For this review, take the finished solid that the model builds, in its own axes (mm). A direction names the side the tool comes from. Coordinates: 2 decimals unless noted, no trailing zeros. Write each loop counter-clockwise with the first axis right and the second up, starting at its lowest first coordinate (ties: lowest second). Pieces come first, ordered by that corner, then holes. Notation, with made-up numbers: M -12.5,44.25 L -1.5,44.25 A18 ccw -1.5,78.25 Z; hole C -2.5,51.25 d9. An arc over 180 degrees is marked long. Return JSON: item names as keys, results as strings.
Autodesk Inventor part; units mm, degrees
ref_plane "YZ Plane" through (0, 0, 0) normal (1, 0, 0) x (0, 1, 0)
ref_plane "XZ Plane" through (0, 0, 0) normal (0, 1, 0) x (-1, 0, 0)
ref_plane "XY Plane" through (0, 0, 0) normal (0, 0, 1) x (1, 0, 0)
sketch "Esquisse1" plane through (0, 0, 0) normal (0, 0, 1) x (1, 0, 0)
  line L0 (-21, -21) -> (21, -21)
  line L1 (21, -21) -> (21, 21)
  line L2 (21, 21) -> (-21, 21)
  line L3 (-21, 21) -> (-21, -21)
  point P0 (0, 0)
  dimension "d0" = 42
  dimension "d1" = 42
  dimension "d2" = 21
  dimension "d3" = 21
extrude "Extrusion1" add sketch "Esquisse1" along normal blind 3
sketch "Esquisse2" plane through (0, 0, 3) normal (0, 0, 1) x (1, 0, 0)
  line L0 (21, 1.8) -> (20, 1.8)
  line L1 (20, 1.8) -> (20, 12.8)
  line L2 (20, 12.8) -> (21, 12.8)
  line L3 (21, 12.8) -> (21, 1.8)
  line L4 (-21, 1.8) -> (-20, 1.8)
  line L5 (-20, 1.8) -> (-20, 12.8)
  line L6 (-20, 12.8) -> (-21, 12.8)
  line L7 (-21, 12.8) -> (-21, 1.8)
  line L8 (21, 21) -> (-21, 21)
  line L9 (-21, 21) -> (-21, -21)
  line L10 (21, -21) -> (21, 21)
  point P0 (0, 0)
  dimension "d6" = 40
  dimension "d7" = 20
  dimension "d8" = 11
  dimension "d9" = 8.2
extrude "Extrusion2" cut sketch "Esquisse2" against normal through all
sketch "Esquisse3" plane through (0, 0, 3) normal (0, 0, 1) x (1, 0, 0)
  line L0 (7.5, 0) -> (7.5, 21)
  line L1 (7.5, 21) -> (-7.5, 21)
  line L2 (-7.5, 21) -> (-7.5, 0)
  line L3 (21, 21) -> (-21, 21)
  arc A0 (-7.5, 0) -> (7.5, 0) centre (0, 0) ccw
  line L4 (-5.5, -11.1) -> (5.5, -11.1) construction
  line L5 (-5.5, -12.6) -> (5.5, -12.6)
  line L6 (5.5, -9.6) -> (-5.5, -9.6)
  arc A1 (-5.5, -9.6) -> (-5.5, -12.6) centre (-5.5, -11.1) ccw
  arc A2 (5.5, -12.6) -> (5.5, -9.6) centre (5.5, -11.1) ccw
  line L7 (-21, -21) -> (21, -21)
  point P0 (0, 0)
  point P1 (0, -11.1)
  dimension "d12" = 15
  dimension "d13" = 7.5
  dimension "d14" = 21
  dimension "d15" = 3
  dimension "d16" = 14
  dimension "d17" = 8.4
extrude "Extrusion3" cut sketch "Esquisse3" against normal through all
sketch "Esquisse4" plane through (0, 0, 0) normal (0, 0, -1) x (-1, 0, 0)
  line L0 (21, -21) -> (-21, -21)
  line L1 (-11, -21) -> (-7.95, -21)
  line L2 (-7.95, -21) -> (-7.95, 21)
  line L3 (-7.95, 21) -> (-11, 21)
  line L4 (-11, 21) -> (-11, -21)
  line L5 (7.95, -21) -> (11, -21)
  line L6 (11, -21) -> (11, 21)
  line L7 (11, 21) -> (7.95, 21)
  line L8 (7.95, 21) -> (7.95, -21)
  line L9 (7.5, 21) -> (21, 21)
  point P0 (0, 0)
  dimension "d20" = 3.05
  dimension "d21" = 3.05
  dimension "d22" = 15.9
  dimension "d23" = 7.95
extrude "Extrusion4" add sketch "Esquisse4" along normal blind 0.5
chamfer "Chanfrein1" distance 0.25 angle 45 12 edges at (16, 21, 0) (21, 16.9, 0) (16, -21, 0) (-16, -21, 0) (-21, -9.6, 0) (-16, 21, 0) (21, -9.6, 0) (-21, 16.9, 3) (-21, -9.6, 3) (0, -21, 3) (21, -9.6, 3) (21, 16.9, 3)
sketch "Esquisse5" plane through (0, 0, 3) normal (0, 0, 1) x (1, 0, 0)
  line L0 (-7.5, 21) -> (-20.75, 21)
  point P0 (0, 0)
  point P1 (-16, 0)
  point P2 (16, 0)
  dimension "d29" = 32
  dimension "d30" = 16
  dimension "d31" = 21
hole "Perçage1" at (-16, 0, 3) at (16, 0, 3) direction (0, 0, -1) diameter 3.5 end through all countersink diameter 6.5 countersink angle 90
equation "\"d21\" = d20"
properties part number "Plaque de maintient" material "----------"
1. We need section A-A (y = -11.1). State the section outline as (x, z) points.
Checks:
{"outline": "M -21,0.25 L -20.75,0 L -11,0 L -11,-0.5 L -7.95,-0.5 L -7.95,0 L -7,0 L -7,3 L -20.75,3 L -21,2.75 Z; M 7,0 L 7.95,0 L 7.95,-0.5 L 11,-0.5 L 11,0 L 20.75,0 L 21,0.25 L 21,2.75 L 20.75,3 L 7,3 Z"}
2. Draft analysis for pull direction Y (two halves, no side actions). For faces 1 (the face through (0, -9.6, 2)), 2 (the face through (-0.16, -7.5, 1.52)), 3 (the face through (14, 0, 0)), state which applies: +Y half, -Y half, draft (parallel to the pull), parting line (faces both ways), or undercut.
Checks:
{"face 1": "undercut", "face 2": "+Y half", "face 3": "draft"}
3. We need section B-B (x = 0). State the section outline as (y, z) points, plus the area to 3 significant figures.
Checks:
{"outline": "M -21,0 L -12.6,0 L -12.6,3 L -20.75,3 L -21,2.75 Z; M -9.6,0 L -7.5,0 L -7.5,3 L -9.6,3 Z", "area": "31.5 mm2"}
4. We need section D-D (x = 16). State the section outline as (y, z) points, plus the area to 3 significant figures.
Checks:
{"outline": "M -21,0.25 L -20.75,0 L -1.75,0 L -1.75,1.5 L -3.25,3 L -20.75,3 L -21,2.75 Z; M 1.75,0 L 20.75,0 L 21,0.25 L 21,3 L 3.25,3 L 1.75,1.5 Z", "area": "113 mm2"}
5. Clearance check with flat-ended pins moving along their axes: pin 1 Ø0.8 at (y, z) = (-1.5, 0) entering from +X; pin 2 Ø8 at (x, y) = (-0.5, -9.5) entering from -Z; pin 3 Ø1.5 at (y, z) = (8, 1.5) entering from -X; pin 4 Ø1.5 at (y, z) = (7.5, 2) entering from +X. State where each tip first meets the part, or that it passes through.
Checks:
{"pin 1": "x = 21", "pin 2": "z = 0", "pin 3": "x = -20", "pin 4": "x = 20"}
6. We need section C-C (z = 2). State the section outline as (x, y) points.
Checks:
{"outline": "M -21,-21 L 21,-21 L 21,1.8 L 20,1.8 L 20,12.8 L 21,12.8 L 21,21 L 7.5,21 L 7.5,0 A7.5 cw -7.5,0 L -7.5,21 L -21,21 L -21,12.8 L -20,12.8 L -20,1.8 L -21,1.8 Z; hole C -16,0 d4.5; hole M -5.5,-12.6 L 5.5,-12.6 A1.5 ccw 5.5,-9.6 L -5.5,-9.6 A1.5 ccw Z; hole C 16,0 d4.5"}
7. For faces 4 (the face through (0, -12.6, 2)), 5 (the face through (-14, 0, 0)), 6 (the face through (7.5, 10, 2)), 7 (the face through (-20, 7, 2)), list the 3-axis set-ups (+Z, -Z, +X, -X, +Y, -Y) from which the entire face can be reached by the end or side of a thin tool; tool diameter is ignored.
Checks:
{"face 4": "+Z, -Z", "face 5": "-Z, -X, +Y, -Y", "face 6": "+Z, -Z, +Y", "face 7": "+Z, -Z, -X"}
8. Wall thickness on L1, parallel to X at y = 0, z = 0.8; L2, parallel to Y at x = -16, z = 0.8; L3, parallel to X at y = 16, z = 2.15: over which ranges is each line inside the solid? List them lowest first. Write a range as from..to.
Checks:
{"L1": "-21..-17.75, -14.25..-7.5, 7.5..14.25, 17.75..21", "L2": "-21..-1.75, 1.75..21", "L3": "-21..-7.5, 7.5..21"}
